from build123d import *

# Parameters (mm, degrees)
SKETCH1_R                   = 46.355
BOSS_EXTRUDE1_DEPTH         = 1.5875
F_1_4_CLEARANCE_HOLE1_D     = 6.7564
F_1_4_CLEARANCE_HOLE1_DEPTH = 48.770172657
F_1_4_CLEARANCE_HOLE1_TIP   = 2.029827343
CUT_EXTRUDE1_DEPTH          = 4.175


with BuildPart() as part:
    # Sketch1 → Boss-Extrude1 (new body, symmetric)
    with BuildSketch(Plane(origin=(0, 0, 0), x_dir=(1, 0, 0), z_dir=(0, 1, 0))):
        Circle(SKETCH1_R)
    extrude(amount=BOSS_EXTRUDE1_DEPTH, both=True)

    # 1/4 Clearance Hole1
    with Locations(Plane(origin=(0, 1.5875, 0), x_dir=(1, 0, 0), z_dir=(0, 1, 0))):
        with Locations((25.4, 0), (-25.4, 0)):
            Hole(F_1_4_CLEARANCE_HOLE1_D / 2, depth=F_1_4_CLEARANCE_HOLE1_DEPTH)
            with Locations((0, 0, -(F_1_4_CLEARANCE_HOLE1_DEPTH + F_1_4_CLEARANCE_HOLE1_TIP / 2))):  # 118° drill point
                Cone(0, F_1_4_CLEARANCE_HOLE1_D / 2, F_1_4_CLEARANCE_HOLE1_TIP, mode=Mode.SUBTRACT)

    # Sketch4 → Cut-Extrude1 (cut, through all)
    with BuildSketch(Plane(origin=(0, 1.5875, 0), x_dir=(1, 0, 0), z_dir=(0, 1, 0))):
        with BuildLine():
            Line((9.525, 9.525), (9.525, -9.525))
            ThreePointArc((9.525, -9.525), (0, -19.05), (-9.525, -9.525))
            Line((-9.525, -9.525), (-9.525, 9.525))
            ThreePointArc((-9.525, 9.525), (0, 19.05), (9.525, 9.525))
        make_face()
    extrude(amount=-CUT_EXTRUDE1_DEPTH, mode=Mode.SUBTRACT)


solid = part.part
Source: CAD feature listing. Evaluate the final solid. Frame: model axes, mm. A direction names the side the tool comes from. Coordinates: 2 decimals unless noted, no trailing zeros. Loops run counter-clockwise (first coordinate to the right, second up) from the corner with the lowest first, then second, coordinate; pieces in that order, holes last. Notation, with made-up numbers: M -20.75,11.25 L 11.25,11.25 A27 cw 11.25,41.25 Z; hole C 88.5,-7 d4. An arc over 180 degrees is marked long. Answer in a Markdown table with one row per item.
Q1. Section C-C on z = 0. Return the cut outline in (x, y) (1 decimal).
Answers below:
| item | result |
|---|---|
| outline | M -46.4,-1.6 L -28.8,-1.6 L -28.8,1.6 L -46.4,1.6 Z; M -22,-1.6 L -9.5,-1.6 L -9.5,1.6 L -22,1.6 Z; M 9.5,-1.6 L 22,-1.6 L 22,1.6 L 9.5,1.6 Z; M 28.8,-1.6 L 46.4,-1.6 L 46.4,1.6 L 28.8,1.6 Z |
Q2. Section B-B on y = 1.1. Return the cut outline in (x, z) (3 decimals), plus the area to 3 significant figures.
Answers below:
| item | result |
|---|---|
| outline | C 0,0 d92.71; hole C -25.4,0 d6.756; hole M -9.525,-9.525 A9.525 ccw 9.525,-9.525 L 9.525,9.525 A9.525 ccw -9.525,9.525 Z; hole C 25.4,0 d6.756 |
| area | 6,030 mm^2 |
Q3. Ray query, probe 1 along X at (y, z) = (-0.95, -14.5); probe 2 along Z at (x, y) = (25.4, -0.1); probe 3 along X at (y, z) = (-0.75, 15.5). Return the intervals inside material, ascending. Write a range as from..to.
Answers below:
| item | result |
|---|---|
| probe 1 | x = -44.03..-8.12, 8.12..44.03 |
| probe 2 | z = -38.78..-3.38, 3.38..38.78 |
| probe 3 | x = -43.69..-7.42, 7.42..43.69 |
Q4. Section D-D on x = 25.4. Return the cut outline in (y, z).
Answers below:
| item | result |
|---|---|
| outline | M -1.59,-38.78 L 1.59,-38.78 L 1.59,-3.38 L -1.59,-3.38 Z; M -1.59,3.38 L 1.59,3.38 L 1.59,38.78 L -1.59,38.78 Z |
Q5. Draft query along X for faces 1 (the cylindrical face through (-22.025, -0.022, -0.149)), 2 (the cylindrical face through (42.8, 0, 17.8)), 3 (the flat face through (10, -1.588, -1)). Return one class per face: pulls with the +X half, pulls with the -X half, needs draft (parallel to the pull), parting line crosses it, or undercut.
Answers below:
| item | result |
|---|---|
| face 1 | undercut |
| face 2 | parting line crosses it |
| face 3 | needs draft |
Q6. First-contact query: pin 1 (1.6 mm diameter, centred on y = 0, z = -1.5, fed in from +X); pin 2 (1.5 mm diameter, centred on y = -0.5, z = -27.5, fed in from -X); pin 3 (1 mm diameter, centred on y = -0.5, z = 17.5, fed in from +X). Flat tips, straight axial feed; report the tip coordinate or a pass-through.
Answers below:
| item | result |
|---|---|
| pin 1 | stops at x = 46.35 |
| pin 2 | stops at x = -37.86 |
| pin 3 | stops at x = 43.13 |
Q7. Set-up query: faces 4 (the flat face through (-9.525, 0, 0)), 5 (the flat face through (10, 1.588, -1)). Return all of +Z, -Z, +X, -X, +Y, -Y with unobstructed straight access to the full face (end or side cutting, diameter ignored); none if empty.
Answers below:
| item | result |
|---|---|
| face 4 | +Y, -Y |
| face 5 | +Z, -Z, +X, -X, +Y |
